Model file for the job. Use its own axes, mm. Face numbers are marked on the shaded views. A direction names the side the tool comes from. Round coordinates to 2 decimals unless told otherwise and drop trailing zeros. Order: outer loops, then holes, each group sorted by start corner. A loop starts at its lowest first (then second) coordinate and runs counter-clockwise, first axis right, second up. Notation, with made-up numbers: (53, -24.75) - (70, -24.75) arc R29 cw to (70, 4.25) - close; hole circle Ø7 at (48, -7.5). An arc over 180 degrees is marked (long way). Put each result on its own line as item: value. Start each with the question number.
Item 1: Saw through at C-C on y = 22. List the corners of the cut face in (x, z), plus the area to 3 significant figures.
Item 2: Mould opens along Y. For the marked faces 4, 5 and 6 say: pulls with the +Y half, pulls with the -Y half, needs draft (parallel to the pull), parting line crosses it, or undercut.
Item 3: Saw through at B-B on x = 31. List the corners of the cut face in (y, z).
Item 4: Probe probe 1 along X at (y, z) = (24.5, 1.25); probe 2 along X at (y, z) = (20.5, 13.75); probe 3 along Z at (x, y) = (31, 3). List the from-to ranges inside material, lowest first.
Item 5: Saw through at A-A on z = 6. List the corners of the cut face in (x, y).
Item 6: Which spindle directions (+Z, -Z, +X, -X, +Y, -Y) get a long thin tool onto all of the face, cutting with end or side? Do the marked faces 1, 2 and 3. Say none if no direction does.
Item 7: Saw through at D-D on x = 9. List the corners of the cut face in (y, z).
Item 8: Pin check, flat tips, straight feed: pin 1 Ø8 at (x, z) = (34.5, 15.5) entering from -Y; pin 2 Ø5 at (x, y) = (13.5, 17) entering from +Z; pin 3 Ø8 at (y, z) = (21.5, 17.5) entering from -X; pin 4 Ø3 at (y, z) = (15.5, 14) entering from +X. Stop position of each tip, or through.
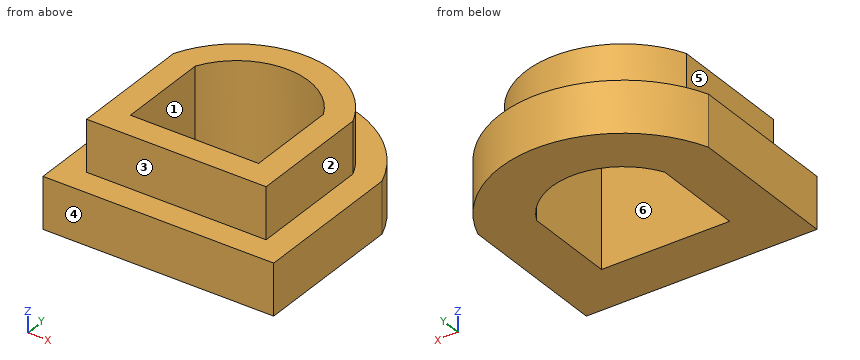
```python
from build123d import *

# Parameters (mm, degrees)
F0_W     = 45
F0_H     = 30
F1_DEPTH = 10
F3_DEPTH = 10
F5_DEPTH = 20


with BuildPart() as f1:
    # F0 (on Top) → F1 (new body)
    with BuildSketch(Plane.XY):
        with Locations((22.5, 15)):
            Rectangle(F0_W, F0_H)
        with BuildLine():
            ThreePointArc((45, 30), (22.5, 45.648353), (0, 30))
            Line((0, 30), (45, 30))
        make_face()
    extrude(amount=F1_DEPTH)

    # F2 (on face) → F3 (join)
    with BuildSketch(Plane.XY.offset(10)):
        with BuildLine():
            Line((5, 5), (40, 5))
            Line((40, 5), (40, 29.047678))
            ThreePointArc((40, 29.047678), (22.5, 40.648353), (5, 29.047678))
            Line((5, 29.047678), (5, 5))
        make_face()
    extrude(amount=F3_DEPTH)

    # F4 (on face) → F5 (cut)
    with BuildSketch(Plane.XY.offset(20)):
        with BuildLine():
            Line((10, 27.953114), (10, 10))
            Line((10, 10), (35, 10))
            Line((35, 10), (35, 27.953114))
            ThreePointArc((35, 27.953114), (22.5, 35.648353), (10, 27.953114))
        make_face()
    extrude(amount=-F5_DEPTH, mode=Mode.SUBTRACT)


solid = f1.part
```
Results found:
1. outline: (0, 0) - (10, 0) - (10, 20) - (5, 20) - (5, 10) - (0, 10) - close; (35, 0) - (45, 0) - (45, 10) - (40, 10) - (40, 20) - (35, 20) - close
1. area: 300 mm²
2. face 4: pulls with the -Y half
2. face 5: needs draft
2. face 6: undercut
3. outline: (0, 0) - (10, 0) - (10, 20) - (5, 20) - (5, 10) - (0, 10) - close; (32.77, 0) - (44.09, 0) - (44.09, 10) - (38.64, 10) - (38.64, 20) - (32.77, 20) - close
4. probe 1: x = 0 to 10, 35 to 45
4. probe 2: x = 5 to 10, 35 to 40
4. probe 3: z = 0 to 10
5. outline: (0, 0) - (45, 0) - (45, 30) arc R24 ccw to (0, 30) - close; hole (10, 10) - (35, 10) - (35, 27.95) arc R14 ccw to (10, 27.95) - close
6. face 1: +Z, -Z
6. face 2: +Z, +X, +Y, -Y
6. face 3: +Z, +X, -X, -Y
7. outline: (0, 0) - (41.49, 0) - (41.49, 10) - (35.02, 10) - (35.02, 20) - (5, 20) - (5, 10) - (0, 10) - close
8. pin 1: stops at y = 5
8. pin 2: passes through
8. pin 3: stops at x = 5
8. pin 4: stops at x = 40
